The model under review builds one solid part; all positions refer to its coordinate system, in mm. Face numbers are marked on the shaded views. Coordinates: 2 decimals unless noted, no trailing zeros. Order: outer loops, then holes, each group sorted by start corner. A loop starts at its lowest first (then second) coordinate and runs counter-clockwise, first axis right, second up. Notation, with made-up numbers: M 57,87.25 L 114,87.25 A24 ccw 114,126.25 Z; hole C -14,8 d8. An arc over 180 degrees is marked long. Answer as CSV lines item,"result". Start each with the question number.
Q1. The part is to be moulded in two halves that separate along Y. For the marked faces 1, 2 and 3, say which applies: +Y half, -Y half, draft (parallel to the pull), parting line (faces both ways), or undercut.
Q2. Wall thickness on L1, parallel to Z at x = 14.95, y = 26.3; L2, parallel to X at y = 9.25, z = -23.73; L3, parallel to Z at x = 6.8, y = 9.5: over which ranges is each line inside the solid? List them lowest first. Write a range as [from, to].
Q3. Consider section C-C on x = 23.75. Write out the cut boundary in (y, z), and give its area (3 significant figures).
Q4. Consider section D-D on z = -23.73. Write out the cut boundary in (x, y).
Q5. Consider section A-A on x = 14.95. Write out the cut boundary in (y, z), and give its area (3 significant figures).
Q6. For P1, Ø2.5, axis at x = 6.8, z = -23.73, coming from the +Y side; P2, Ø8, axis at y = 24.5, z = -14.5, coming from the -X side, all flat-tipped, find the tip position at first contact; note any pin that passes through.
Q7. Consider section B-B on y = 13.25. Write out the cut boundary in (x, z), and give its area (3 significant figures).
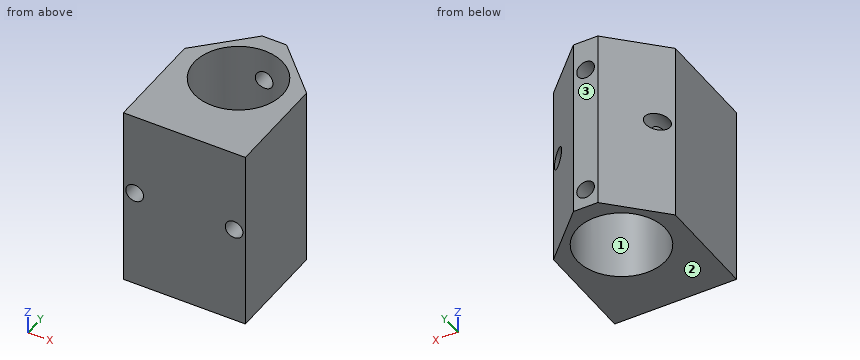
Autodesk Inventor part; units mm, degrees
ref_plane "YZ Plane" through (0, 0, 0) normal (1, 0, 0) x (0, 1, 0)
ref_plane "XZ Plane" through (0, 0, 0) normal (0, 1, 0) x (-1, 0, 0)
ref_plane "XY Plane" through (0, 0, 0) normal (0, 0, 1) x (1, 0, 0)
ref_plane "Work Plane1" through (0, 0, 0) normal (0, 0, 1) x (1, 0, 0)
ref_plane "Work Plane2" through (0, 0, -10) normal (0, 0, 1) x (1, 0, 0)
sketch "Sketch1" plane through (0, 0, -10) normal (0, 0, 1) x (1, 0, 0)
  circle A0 centre (14.95, 17.4977) radius 7.15
  line L0 (0, 2.471) -> (29.9, 2.471)
  line L1 (0, 2.471) -> (0, 18.471)
  line L2 (0, 18.471) -> (-2, 18.471)
  line L3 (-2, 18.471) -> (-2, -1.5)
  line L4 (29.9, -1.5) -> (-2, -1.5)
  line L5 (29.9, -1.5) -> (29.9, 2.471)
  line L6 (4.95, 2.471) -> (24.95, 2.471)
  line L7 (24.95, 2.471) -> (24.95, 27.471)
  line L8 (24.95, 27.471) -> (4.95, 27.471)
  line L9 (4.95, 27.471) -> (4.95, 2.471)
  circle A1 centre (14.95, 17.4977) radius 7.25
  point P0 (0, 0)
  dimension "d6" = 20
  dimension "d7" = 25
  dimension "d8" = 10
  dimension "d9" = 0.1
extrude "Extrusion1" add sketch "Sketch1" against normal blind 30 contours L9 L8 L7 L0
sketch "Sketch2" plane through (4.95, 2.471, -10) normal (0, -1, 0) x (1, 0, 0)
  circle A0 centre (18.15, -13.73) radius 2.45
  circle A1 centre (1.85, -13.73) radius 2.75
  circle A2 centre (18.15, -13.73) radius 1.45
  circle A3 centre (1.85, -13.73) radius 1.45
  point P0 (-4.95, 10)
  dimension "d10" = 2.9
  dimension "d11" = 2.9
extrude "Extrusion2" cut sketch "Sketch2" against normal through all contours A2 | A3
chamfer "Chamfer1" distance 8 angle 45 2 edges at (24.95, 27.471, -25) (4.95, 27.471, -25)
sketch "Sketch3" plane through (12.95, 27.471, -10) normal (0, 1, 0) x (1, 0, 0)
  line L0 (0, 0) -> (0, 30)
  line L1 (4, 0) -> (0, 0)
  line L2 (4, 30) -> (4, 0)
  line L3 (0, 30) -> (4, 30)
  circle A0 centre (2, 5.2757) radius 1.45
  circle A1 centre (2, 26.8475) radius 1.45
  point P0 (-12.95, -10)
  dimension "d17" = 2.9
  dimension "d18" = 2.9
extrude "Extrusion3" cut sketch "Sketch3" against normal blind 10 contours A0 | A1
ref_plane "Work Plane3" through (0, 27.471, -10) normal (0, -0.7071068, 0.7071068) x (1, 0, 0)
ref_plane "Work Plane4" through (12.95, 27.471, -10) normal (0, 0.7071068, 0.7071068) x (1, 0, 0)
ref_plane "Work Plane5" through (14.95, 2.471, -10) normal (1, 0, 0) x (0, 0, -1)
sketch "Sketch5" plane through (14.95, 2.471, -10) normal (1, 0, 0) x (0, 0, -1)
  line L0 (0, 22.2768) -> (30, 22.2768)
  line L1 (0, 7.7768) -> (30, 7.7768)
  line L2 (0, 22.2768) -> (-4.2183, 22.2768)
  line L3 (-4.2183, 22.2768) -> (24.7731, 51.2681)
  line L4 (24.7731, 51.2681) -> (24.7731, 22.2768)
  point P0 (-10, -2.471)
  dimension "d21" = 41
  dimension "d22" = 45
properties part number "cellSTORM_v5_greenlaser_adapter"
Evaluation:
1,face 1,"undercut"
1,face 2,"draft"
1,face 3,"+Y half"
2,L1,"z = [-40, -38.3], [-35.4, -16.73], [-13.83, -10]"
2,L2,"x = [4.95, 5.35], [8.25, 21.65], [24.55, 24.95]"
2,L3,"z = [-40, -25.18], [-22.28, -10]"
3,outline,"M 2.47,-40 L 20.67,-40 L 20.67,-25.03 L 2.47,-25.03 Z; M 2.47,-22.43 L 20.67,-22.43 L 20.67,-10 L 2.47,-10 Z"
3,area,"499 mm²"
4,outline,"M 4.95,2.47 L 5.35,2.47 L 5.35,19.87 L 4.95,19.47 Z; M 8.25,2.47 L 21.65,2.47 L 21.65,14.73 A7.25 cw 8.25,14.73 Z; M 8.25,20.27 A7.25 cw 21.65,20.27 L 21.65,22.77 L 16.95,27.47 L 12.95,27.47 L 8.25,22.77 Z; M 24.55,2.47 L 24.95,2.47 L 24.95,19.47 L 24.55,19.87 Z"
5,outline,"M 2.47,-40 L 10.25,-40 L 10.25,-10 L 2.47,-10 Z; M 24.75,-40 L 27.47,-40 L 27.47,-38.3 L 24.75,-38.3 Z; M 24.75,-35.4 L 27.47,-35.4 L 27.47,-16.73 L 24.75,-16.73 Z; M 24.75,-13.83 L 27.47,-13.83 L 27.47,-10 L 24.75,-10 Z"
5,area,"299 mm²"
6,P1,"passes through"
6,P2,"stops at x = 5.98"
7,outline,"M 4.95,-40 L 9.07,-40 L 9.07,-10 L 4.95,-10 Z; M 20.83,-40 L 24.95,-40 L 24.95,-10 L 20.83,-10 Z; hole C 6.8,-23.73 d2.9; hole C 23.1,-23.73 d2.9"
7,area,"234 mm²"
